Could you check a few things on this drawing? It's one solid part, dimensions in mm from its lowest x, y, z. A direction names the side the tool comes from. Round coordinates to 2 decimals unless told otherwise and drop trailing zeros. Write each loop counter-clockwise with the first axis right and the second up, starting at its lowest first coordinate (ties: lowest second). Pieces come first, ordered by that corner, then holes. Notation, with made-up numbers: (35.25, 49.5) - (69.25, 49.5) arc R10 ccw to (69.25, 54.5) - close; hole circle Ø3 at (86.25, -8). An arc over 180 degrees is marked (long way). Use one line per item in the form item = value. Start each with the question number.
1. I want a section at D-D, the plane x = 356. List the corners of the cut face in (y, z) for me, plus the area to 3 significant figures.
2. If I drill on line 1 along Y through (x, z) = (162.5, 5); line 2 along X through (y, z) = (23, 24.5); line 3 along Y through (x, z) = (52.5, 91), over which ranges is the centre line in solid material (lowest first)?
3. Will these pins go through, and if not, where does the flat tip stop? pin 1 (11.5 mm diameter, centred on y = 26, z = 121, fed in from +X); pin 2 (19 mm diameter, centred on y = 12.5, z = 59, fed in from -X); pin 3 (5 mm diameter, centred on x = 286.5, y = 48, fed in from +Z).
4. I want a section at B-B, the plane y = 48.5. List the corners of the cut face in (x, z) for me, plus the area to 3 significant figures.
5. I want a section at C-C, the plane z = 106. List the corners of the cut face in (x, y) for me (1 decimal).
6. We'd pull the mould along X, two halves only. Please class the marked faces 1, 2 and 3: +X half, -X half, draft (parallel to the pull), parting line (faces both ways), or undercut.
7. Which directions (+Z, -Z, +X, -X, +Y, -Y) give clear straight access to the entire face, cutting with the end or side of a thin tool? Please do the marked faces 4, 5 and 6.
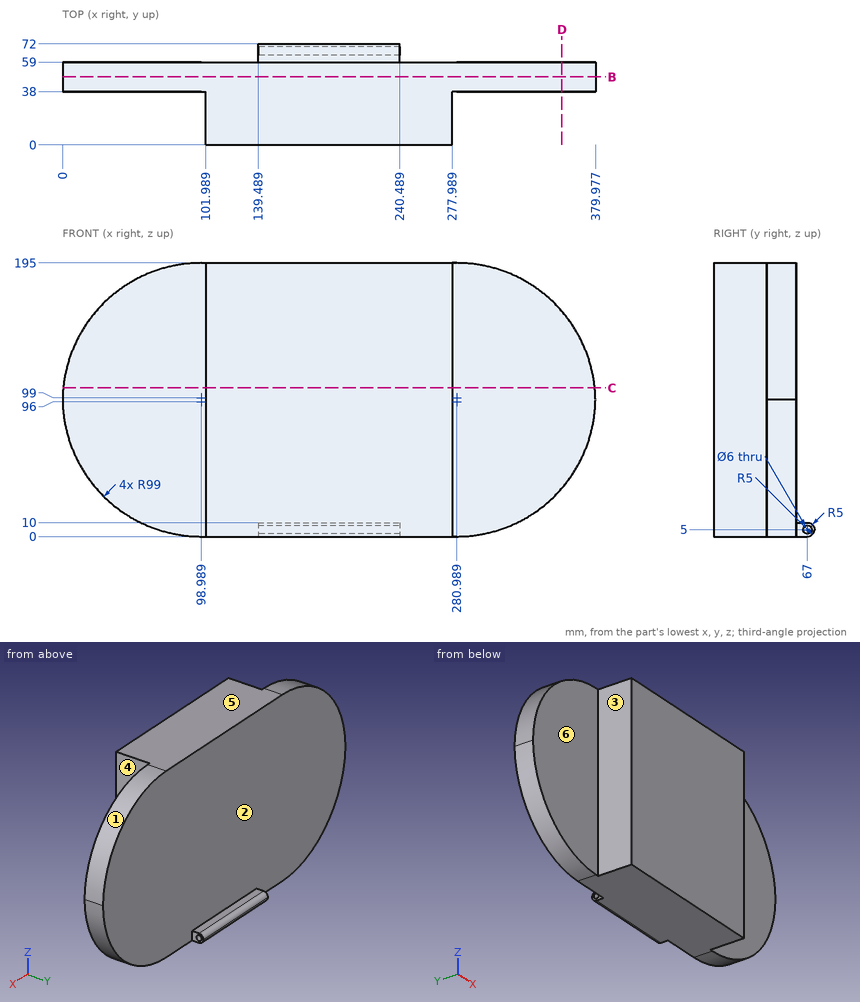
Model answer:
q1.outline = (38, 34.39) - (59, 34.39) - (59, 160.61) - (38, 160.61) - close
q1.area = 2,650 mm2
q2.line_1 = 0 to 64, 70 to 72
q2.line_2 = 101.99 to 277.99
q2.line_3 = 38 to 59
q3.pin_1 = 277.99
q3.pin_2 = 101.99
q3.pin_3 = 194.95
q4.outline = (0, 97.5) arc R99 ccw to (98.99, 0) - (280.99, 0) arc R99 ccw to (379.98, 97.5) arc R99 ccw to (280.99, 195) - (98.99, 195) arc R99 ccw to start
q4.area = 65,700 mm2
q5.outline = (0.5, 38) - (102, 38) - (102, 0) - (278, 0) - (278, 38) - (379.5, 38) - (379.5, 59) - (0.5, 59) - close
q6.face_1 = +X half
q6.face_2 = draft
q6.face_3 = -X half
q7.face_4 = +Z, -Z, +X, -Y
q7.face_5 = +Z, +X, -X, +Y, -Y
q7.face_6 = +Z, -Z, -X, -Y
